The listing builds one solid part. Answer for the finished solid, in the listing's coordinates (mm). Give positions to 0.01 mm unless a question says otherwise; leave off trailing zeros. Loops run counter-clockwise (first coordinate to the right, second up) from the corner with the lowest first, then second, coordinate; pieces in that order, holes last. Notation, with made-up numbers: M 46.5,39.5 L 102.5,39.5 A19 cw 102.5,72.5 Z; hole C -24.5,66.5 d9. An arc over 180 degrees is marked long. One line per item, written item: value. Start each with the question number.
Q1. A cutting plane is placed at A-A, the plane z = 0. Determine the outline of the cut face in (x, y).
Q2. A cutting plane is placed at D-D, the plane x = 45.5. Determine the outline of the cut face in (y, z), and give its area (3 significant figures).
Q3. A cutting plane is placed at B-B, the plane x = -45. Determine the outline of the cut face in (y, z).
Q4. A cutting plane is placed at C-C, the plane y = 2.1. State how many separate pieces and enclosed holes the cut face has, and give its area (3 significant figures).
Q5. Consider L1, parallel to X at y = 2, z = 0; L2, parallel to Z at x = -45, y = 2.25; L3, parallel to X at y = 1.05, z = -25. Determine where each line is inside the solid, lowest interval first.
Q6. Flat-ended cylindrical pins translate along their axes: pin 1 (0.9 mm diameter, centred on x = 57.5, y = 2, fed in from +Z); pin 2 (1.5 mm diameter, centred on y = 1, z = 65, fed in from +X); pin 3 (1.5 mm diameter, centred on x = -64.5, y = 1.5, fed in from -Z). Find the tip coordinate at first contact, or state that the pin passes through.
from build123d import *

# Parameters (mm, degrees)
BOSS_EXTRUDE1_DEPTH = 3
SKETCH4_R           = 3
CUT_EXTRUDE2_DEPTH  = 16


with BuildPart() as part:
    # Sketch1 → Boss-Extrude1 (new body)
    with BuildSketch(Plane(origin=(0, 0, 0), x_dir=(1, 0, 0), z_dir=(0, 1, 0))):
        Polygon((7.5, -62.5), (7.5, -66.5), (22.5, -66.5), (22.5, -62.5), (32.5, -62.5), (32.5, -66.5), (47.5, -66.5), (47.5, -62.5), (57.5, -62.5), (62.5, -62.5), (62.5, -59), (62.5, -47.5), (66.5, -47.5), (66.5, -32.5), (62.5, -32.5), (62.5, -22.5), (66.5, -22.5), (66.5, -7.5), (62.5, -7.5), (62.5, 7.5), (66.5, 7.5), (66.5, 22.5), (62.5, 22.5), (62.5, 32.5), (66.5, 32.5), (66.5, 47.5), (62.5, 47.5), (62.5, 59), (62.5, 62.5), (57.5, 62.5), (47.5, 62.5), (47.5, 66.5), (32.5, 66.5), (32.5, 62.5), (22.5, 62.5), (22.5, 66.5), (7.5, 66.5), (7.5, 62.5), (-7.5, 62.5), (-7.5, 66.5), (-22.5, 66.5), (-22.5, 62.5), (-32.5, 62.5), (-32.5, 66.5), (-47.5, 66.5), (-47.5, 62.5), (-59, 62.5), (-62.5, 62.5), (-62.5, 59), (-62.5, 47.5), (-66.5, 47.5), (-66.5, 32.5), (-62.5, 32.5), (-62.5, 22.5), (-66.5, 22.5), (-66.5, 7.5), (-62.5, 7.5), (-62.5, -7.5), (-66.5, -7.5), (-66.5, -22.5), (-62.5, -22.5), (-62.5, -32.5), (-66.5, -32.5), (-66.5, -47.5), (-62.5, -47.5), (-62.5, -59), (-62.5, -62.5), (-59, -62.5), (-47.5, -62.5), (-47.5, -66.5), (-32.5, -66.5), (-32.5, -62.5), (-22.5, -62.5), (-22.5, -66.5), (-7.5, -66.5), (-7.5, -62.5), align=None)
    extrude(amount=BOSS_EXTRUDE1_DEPTH)

    # Sketch4 → Cut-Extrude2 (cut)
    with BuildSketch(Plane(origin=(0, 0, 0), x_dir=(1, 0, 0), z_dir=(0, 1, 0))):
        with Locations((-45, 0)):
            Circle(SKETCH4_R)
        with Locations((45, 0)):
            Circle(SKETCH4_R)
    extrude(amount=CUT_EXTRUDE2_DEPTH, mode=Mode.SUBTRACT)


solid = part.part
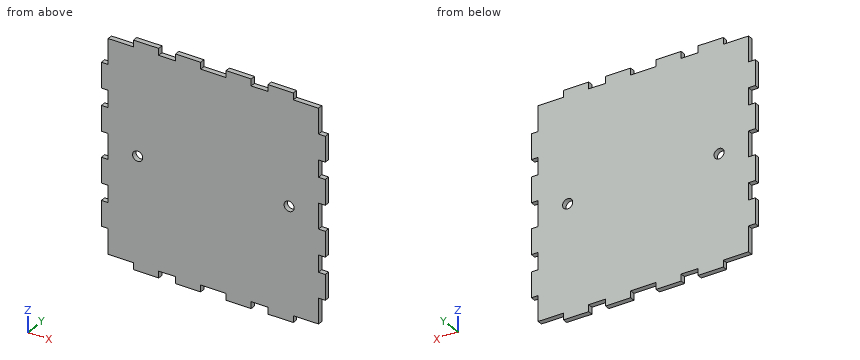
Answer block:
1. outline: M -62.5,0 L -48,0 L -48,3 L -62.5,3 Z; M -42,0 L 42,0 L 42,3 L -42,3 Z; M 48,0 L 62.5,0 L 62.5,3 L 48,3 Z
2. outline: M 0,-66.5 L 3,-66.5 L 3,-2.96 L 0,-2.96 Z; M 0,2.96 L 3,2.96 L 3,66.5 L 0,66.5 Z
2. area: 381 mm^2
3. outline: M 0,-66.5 L 3,-66.5 L 3,-3 L 0,-3 Z; M 0,3 L 3,3 L 3,66.5 L 0,66.5 Z
4. separate pieces: 1
4. enclosed holes: 2
4. area: 16,500 mm^2
5. L1: -62.5 to -48, -42 to 42, 48 to 62.5
5. L2: -66.5 to -3, 3 to 66.5
5. L3: -62.5 to 62.5
6. pin 1: z = 62.5
6. pin 2: x = 47.5
6. pin 3: z = -47.5
